```python
from build123d import *

# Parameters (mm, degrees)
SKETCH1_R            = 1
BOSS_EXTRUDE1_DEPTH  = 1.2
FILLET1_R            = 2.07
FILLET4_R            = 0.52
FILLET1_OF_MIRROR1_R = 2.07
FILLET4_OF_MIRROR1_R = 0.52


with BuildPart() as part:
    # Sketch1 → Boss-Extrude1 (new body)
    with BuildSketch(Plane.XY):
        with BuildLine():
            Line((0, 10.716160966), (0, 8.316160966))
            ThreePointArc((0, 8.316160966), (-8.248743485, 0.21014332), (-0.287920848, -8.178813356))
            Line((-0.287920848, -8.178813356), (-0.424287349, -12.083839034))
            ThreePointArc((-0.424287349, -12.083839034), (-2.896253939, -11.741219474), (-5.246180053, -10.901068155))
            Line((-5.246180053, -10.901068155), (-5.359136951, -7.71729271))
            ThreePointArc((-5.359136951, -7.71729271), (-9.598340525, 3.51092083), (0, 10.716160966))
        make_face()
        with Locations((-2.430824062, -9.84376582)):
            Circle(SKETCH1_R, mode=Mode.SUBTRACT)
    boss_extrude1 = extrude(amount=BOSS_EXTRUDE1_DEPTH)

    # Fillet1
    fillet1_edges = [part.edges().sort_by_distance(p)[0] for p in [
        (-5.359136951, -7.71729271, 0.6),
    ]]
    fillet(fillet1_edges, radius=FILLET1_R)

    # Fillet4
    fillet4_edges = [part.edges().sort_by_distance(p)[0] for p in [
        (-5.246180053, -10.901068155, 0.6),
    ]]
    fillet(fillet4_edges, radius=FILLET4_R)

    # Mirror1: Boss-Extrude1 across plane
    add(boss_extrude1.mirror(Plane(origin=(0, 10.716160966, 1.2), x_dir=(0, 0, 1), z_dir=(-1, 0, 0))))

    # Fillet1 of Mirror1
    fillet1_of_mirror1_edges = [part.edges().sort_by_distance(p)[0] for p in [
        (5.359136951, -7.71729271, 0.6),
    ]]
    fillet(fillet1_of_mirror1_edges, radius=FILLET1_OF_MIRROR1_R)

    # Fillet4 of Mirror1
    fillet4_of_mirror1_edges = [part.edges().sort_by_distance(p)[0] for p in [
        (5.246180053, -10.901068155, 0.6),
    ]]
    fillet(fillet4_of_mirror1_edges, radius=FILLET4_OF_MIRROR1_R)


solid = part.part
```
Verification items for the finished model (mm, model axes). Give positions to 0.01 mm unless a question says otherwise; leave off trailing zeros. Order: outer loops, then holes, each group sorted by start corner. A loop starts at its lowest first (then second) coordinate and runs counter-clockwise, first axis right, second up. Notation, with made-up numbers: (-19.5, 84.25) -> (-15.5, 84.25) arc R21 cw to (-15.5, 108.25) -> close; hole circle Ø9 at (25, 69). An arc over 180 degrees is marked (long way). One line per item, written item: value.
(1) Sectioned sample at C-C on z = 0.65. Record the cut outline in (x, y), then the cut area to 3 significant figures.
Final values:
outline: (-6.12, -7.18) arc R2.07 cw to (-5.32, -8.74) -> (-5.26, -10.58) arc R0.52 ccw to (-4.95, -11.04) arc R12.16 ccw to (-0.42, -12.08) -> (-0.29, -8.18) arc R8.25 cw (long way) to (0.29, -8.18) -> (0.42, -12.08) arc R12.16 ccw to (4.95, -11.04) arc R0.52 ccw to (5.26, -10.58) -> (5.32, -8.74) arc R2.07 cw to (6.12, -7.18) arc R10 ccw (long way) to start; hole circle Ø2 at (-2.43, -9.84); hole circle Ø2 at (2.43, -9.84)
area: 122 mm^2
(2) Scan lines: line 1 along Y through (x, z) = (3.25, 0.55); line 2 along Y through (x, z) = (-1.75, 0.4); line 3 along Y through (x, z) = (-4.5, 0.75). Record each from-to range of solid material in increasing order. Write a range as [from, to].
Final values:
line 1: [-11.65, -10.42], [-9.27, -7.52], [7.65, 10.17]
line 2: [-11.96, -10.58], [-9.11, -8], [8.13, 10.56]
line 3: [-11.23, -6.85], [6.98, 9.65]
(3) Sectioned sample at A-A on y = 1.25. Record the cut outline in (x, z), then the cut area to 3 significant figures.
Final values:
outline: (-9.98, 0) -> (-8.16, 0) -> (-8.16, 1.2) -> (-9.98, 1.2) -> close; (8.16, 0) -> (9.98, 0) -> (9.98, 1.2) -> (8.16, 1.2) -> close
area: 4.36 mm^2
(4) Sectioned sample at D-D on x = 1. Record the cut outline in (y, z), then the cut area to 3 significant figures.
Final values:
outline: (-12.05, 0) -> (-8.12, 0) -> (-8.12, 1.2) -> (-12.05, 1.2) -> close; (8.26, 0) -> (10.67, 0) -> (10.67, 1.2) -> (8.26, 1.2) -> close
area: 7.61 mm^2
(5) Sectioned sample at B-B on x = -3. Record the cut outline in (y, z), then the cut area to 3 significant figures.
Final values:
outline: (-11.72, 0) -> (-10.67, 0) -> (-10.67, 1.2) -> (-11.72, 1.2) -> close; (-9.02, 0) -> (-7.62, 0) -> (-7.62, 1.2) -> (-9.02, 1.2) -> close; (7.75, 0) -> (10.26, 0) -> (10.26, 1.2) -> (7.75, 1.2) -> close
area: 5.95 mm^2
